from build123d import *

# Parameters (mm, degrees)
ESQUISSE1_R                  = 10.25
BOSS_EXTRU_1_DEPTH           = 1
D_GAGEMENT_M21_D             = 2.6
R_P_TITION_CIRCULAIRE1_COUNT = 4
ESQUISSE9_R                  = 5.5
BOSS_EXTRU_4_DEPTH           = 8
ENL_V_MAT_EXTRU_1_DEPTH      = 6
CONG_1_R                     = 0.5


with BuildPart() as part:
    # Esquisse1 → Boss.-Extru.1 (new body)
    with BuildSketch(Plane.XZ.offset(38.601290575)):
        with Locations(Location((14.017249305, 17.25, 0), (0, 0, 270))):
            Circle(ESQUISSE1_R)
    extrude(amount=BOSS_EXTRU_1_DEPTH)

    # Dégagement M21 (through all)
    with Locations(Plane(origin=(0, -39.601290575, 0), x_dir=(-1, 0, 0), z_dir=(0, -1, 0))):
        with Locations((-11.415520349, -24.815117741)):
            d_gagement_m21 = Hole(D_GAGEMENT_M21_D / 2)

    # Répétition circulaire1: Dégagement M21 ×4 about axis
    r_p_tition_circulaire1_axis = Axis((14.017249305, 0, 17.25), (0, 1, 0))
    for i in range(1, R_P_TITION_CIRCULAIRE1_COUNT):
        add(d_gagement_m21.rotate(r_p_tition_circulaire1_axis, i * 360 / R_P_TITION_CIRCULAIRE1_COUNT), mode=Mode.SUBTRACT)

    # Esquisse9 → Boss.-Extru.4 (add)
    with BuildSketch(Plane(origin=(0, -39.601290575, 0), x_dir=(-1, 0, 0), z_dir=(0, -1, 0))):
        with Locations(Location((-14.017249305, -17.25, 0), (0, 0, 90))):
            Circle(ESQUISSE9_R)
    extrude(amount=BOSS_EXTRU_4_DEPTH)

    # Esquisse10 → Enlèv. mat.-Extru.1 (cut)
    with BuildSketch(Plane.XZ.offset(47.601290575)):
        with BuildLine():
            Line((11.904786288, 19.85), (16.129712323, 19.85))
            ThreePointArc((16.129712323, 19.85), (14.017249305, 13.9), (11.904786288, 19.85))
        make_face()
    extrude(amount=-ENL_V_MAT_EXTRU_1_DEPTH, mode=Mode.SUBTRACT)

    # Congé1
    cong_1_edges = [part.edges().sort_by_distance(p)[0] for p in [
        (14.017249305, -39.601290575, 22.75),
    ]]
    fillet(cong_1_edges, radius=CONG_1_R)


solid = part.part
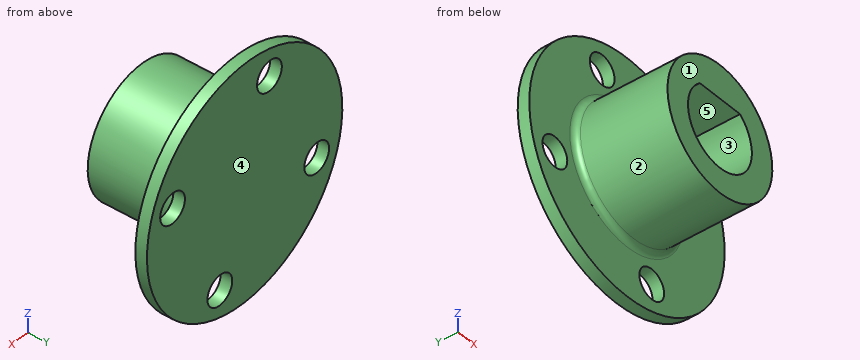
The listing builds one solid part. Answer for the finished solid, in the listing's coordinates (mm). Face numbers are marked on the shaded views. A direction names the side the tool comes from. Round coordinates to 2 decimals unless told otherwise and drop trailing zeros. Write each loop counter-clockwise with the first axis right and the second up, starting at its lowest first coordinate (ties: lowest second). Pieces come first, ordered by that corner, then holes. Notation, with made-up numbers: (30, 26) - (65, 26) arc R25 ccw to (65, 64) - close; hole circle Ø9 at (-38.75, 46). An arc over 180 degrees is marked (long way). Use a Markdown table: item, result. Add a question column.
1. Flat-ended cylindrical pins translate along their axes: P1, Ø3.5, axis at x = 16.62, z = 9.68, coming from the -Y side; P2, Ø2, axis at x = 9.5, y = -43, coming from the +Z side; P3, Ø6, axis at x = 16.5, z = 19, coming from the -Y side; P4, Ø5, axis at y = -45.5, z = 22, coming from the +X side. Find the tip coordinate at first contact, or state that the pin passes through.
2. The part is cut by section A-A (z = 17.25). Write down the section's boundary in (x, y).
3. The part is cut by section B-B (x = 6). Write down the section's boundary in (y, z), and give its area (3 significant figures).
4. A tool of negligible diameter and unlimited length cuts with its end or side. For the marked faces 4 and 5, from which of +Z, -Z, +X, -X, +Y, -Y can it reach the whole face along a straight path? Write none if from no direction.
5. For a pull along Z with two mould halves and no side action, classify the marked faces 1, 2 and 3 as +Z half, -Z half, draft (parallel to the pull), parting line (faces both ways), or undercut.
6. The part is cut by section D-D (y = -41.25). Write down the section's boundary in (x, z).
7. Consider line 1 (X direction, y = -44.7, z = 17.25); line 2 (Y direction, x = 14, z = 8.75); line 3 (Z direction, x = 15.75, y = -39.5). Determine where each line is inside the solid, lowest interval first.
8. The part is cut by section C-C (y = -42.75). Write down the section's boundary in (x, z), and give its area (3 significant figures).
Reported:
| question | item | result |
|---|---|---|
| 1 | P1 | y = -39.6 |
| 1 | P2 | z = 21.48 |
| 1 | P3 | y = -47.6 |
| 1 | P4 | x = 19.04 |
| 2 | outline | (3.77, -39.6) - (8.02, -39.6) arc R0.5 cw to (8.52, -40.1) - (8.52, -47.6) - (10.67, -47.6) - (10.67, -41.6) - (17.37, -41.6) - (17.37, -47.6) - (19.52, -47.6) - (19.52, -40.1) arc R0.5 cw to (20.02, -39.6) - (24.27, -39.6) - (24.27, -38.6) - (3.77, -38.6) - close |
| 3 | outline | (-39.6, 10.86) - (-38.6, 10.86) - (-38.6, 13.43) - (-39.6, 13.43) - close; (-39.6, 15.87) - (-38.6, 15.87) - (-38.6, 23.64) - (-39.6, 23.64) - close |
| 3 | area | 10.3 mm^2 |
| 4 | face 4 | +Z, -Z, +X, -X, +Y |
| 4 | face 5 | -Y |
| 5 | face 1 | draft |
| 5 | face 2 | parting line |
| 5 | face 3 | undercut |
| 6 | outline | circle Ø11 at (14.02, 17.25) |
| 7 | line 1 | 8.52 to 10.67, 17.37 to 19.52 |
| 7 | line 2 | -39.6 to -38.6 |
| 7 | line 3 | 7.15 to 8.72, 10.65 to 27.35 |
| 8 | outline | circle Ø11 at (14.02, 17.25); hole (11.9, 19.85) arc R3.35 ccw (long way) to (16.13, 19.85) - close |
| 8 | area | 61.9 mm^2 |
